The model under review builds one solid part; all positions refer to its coordinate system, in mm. A direction names the side the tool comes from. Give positions to 0.01 mm unless a question says otherwise; leave off trailing zeros. Loops run counter-clockwise (first coordinate to the right, second up) from the corner with the lowest first, then second, coordinate; pieces in that order, holes last. Notation, with made-up numbers: M -14,3.25 L 34,3.25 A15 cw 34,12.25 Z; hole C 39.5,77.5 d6. An arc over 180 degrees is marked long. Return JSON: item names as keys, results as strings.
```python
from build123d import *

# Parameters (mm, degrees)
BOSS_EXTRUDE1_DEPTH  = 10
FILLET1_R            = 1
SKETCH2_W            = 21.86553483
SKETCH2_H            = 30.5
CUT_EXTRUDE1_DEPTH   = 5
FILLET1_OF_MIRROR1_R = 1


with BuildPart() as part:
    # Sketch1 → Boss-Extrude1 (new body)
    with BuildSketch(Plane(origin=(0, 0, 0), x_dir=(1, 0, 0), z_dir=(0, 1, 0))):
        Polygon((-5, 57.097150921), (34.3, 57.097150921), (34.3, 55.097150921), (31.675, 55.097150921), (31.675, 52.597150921), (31.675, 2.599340873), (31.675, 0.099340873), (34.3, 0.099340873), (34.3, -4.5), (-5, -4.5), align=None)
        Polygon((-2.625, 45), (-2.625, 0), (-2.625, -2.5), (0, -2.5), (2.625, -2.5), (2.625, 0), (2.625, 45), (2.625, 47.5), (0, 47.5), (-2.625, 47.5), align=None, mode=Mode.SUBTRACT)
    boss_extrude1 = extrude(amount=BOSS_EXTRUDE1_DEPTH)

    # Fillet1
    fillet1_edges = [part.edges().sort_by_distance(p)[0] for p in [
        (31.675, 5, -55.097150921),
        (31.675, 5, -0.099340873),
        (-2.625, 5, -47.5),
        (-2.625, 5, 2.5),
        (2.625, 5, 2.5),
        (2.625, 5, -47.5),
    ]]
    fillet(fillet1_edges, radius=FILLET1_R)

    # Sketch2 → Cut-Extrude1 (cut)
    with BuildSketch(Plane(origin=(0, 10, 0), x_dir=(1, 0, 0), z_dir=(0, 1, 0))):
        with Locations((20.742232585, 23.8519351)):
            Rectangle(SKETCH2_W, SKETCH2_H)
    cut_extrude1 = extrude(amount=-CUT_EXTRUDE1_DEPTH, mode=Mode.SUBTRACT)

    # Mirror1: Boss-Extrude1, Cut-Extrude1 across plane
    add(boss_extrude1.mirror(Plane(origin=(34.3, 10, -0.099340873), x_dir=(0, 0, 1), z_dir=(-1, 0, 0))))
    add(cut_extrude1.mirror(Plane(origin=(34.3, 10, -0.099340873), x_dir=(0, 0, 1), z_dir=(-1, 0, 0))), mode=Mode.SUBTRACT)

    # Fillet1 of Mirror1
    fillet1_of_mirror1_edges = [part.edges().sort_by_distance(p)[0] for p in [
        (36.925, 5, -55.097150921),
        (36.925, 5, -0.099340873),
        (71.225, 5, -47.5),
        (71.225, 5, 2.5),
        (65.975, 5, 2.5),
        (65.975, 5, -47.5),
    ]]
    fillet(fillet1_of_mirror1_edges, radius=FILLET1_OF_MIRROR1_R)


solid = part.part
```
1) Wall thickness on L1, parallel to X at y = 8, z = -14.5 (3 decimals); L2, parallel to X at y = 4.75, z = -46 (3 decimals); L3, parallel to X at y = 9.75, z = 1 (3 decimals): over which ranges is each line inside the solid? List them lowest first. Write a range as from..to.
From the geometry:
{"L1": "-5..-2.625, 2.625..9.809, 58.791..65.975, 71.225..73.6", "L2": "-5..-2.625, 2.625..31.675, 36.925..65.975, 71.225..73.6", "L3": "-5..-2.625, 2.625..65.975, 71.225..73.6"}
2) The part is to be moulded in two halves that separate along Z. For faces 1 (the face through (2.625, 5, -23)), 2 (the face through (42, 0, -27)), 3 (the face through (34, 5, 4.5)), say which applies: released by +Z, released by -Z, zero draft, split by the parting line, or undercut.
From the geometry:
{"face 1": "undercut", "face 2": "zero draft", "face 3": "released by +Z"}
3) Insertion check: pin 1 (1 mm diameter, centred on x = 32, z = -22.5, fed in from +Y). The pin has a flat end and moves straight along its axis. Give the tip position at first contact, or say it passes through.
From the geometry:
{"pin 1": "y = 5"}
4) Consider section A-A on x = 0.5. Write out the cut boundary in (y, z).
From the geometry:
{"outline": "M 0,-57.1 L 10,-57.1 L 10,-47.5 L 0,-47.5 Z; M 0,2.5 L 10,2.5 L 10,4.5 L 0,4.5 Z"}
5) Consider section B-B on z = -36. Write out the cut boundary in (x, y) (3 decimals), then the cut area to 3 significant figures.
From the geometry:
{"outline": "M -5,0 L -2.625,0 L -2.625,10 L -5,10 Z; M 2.625,0 L 31.675,0 L 31.675,5 L 9.809,5 L 9.809,10 L 2.625,10 Z; M 36.925,0 L 65.975,0 L 65.975,10 L 58.791,10 L 58.791,5 L 36.925,5 Z; M 71.225,0 L 73.6,0 L 73.6,10 L 71.225,10 Z", "area": "410 mm²"}
6) Consider section D-D on y = 4. Write out the cut boundary in (x, z) (3 decimals), then the cut area to 3 significant figures.
From the geometry:
{"outline": "M -5,-57.097 L 73.6,-57.097 L 73.6,4.5 L -5,4.5 Z; hole M -2.625,-46.5 A1 ccw -1.625,-47.5 L 1.625,-47.5 A1 ccw 2.625,-46.5 L 2.625,1.5 A1 ccw 1.625,2.5 L -1.625,2.5 A1 ccw -2.625,1.5 Z; hole M 31.675,-54.097 A1 ccw 32.675,-55.097 L 35.925,-55.097 A1 ccw 36.925,-54.097 L 36.925,-1.099 A1 ccw 35.925,-0.099 L 32.675,-0.099 A1 ccw 31.675,-1.099 Z; hole M 65.975,-46.5 A1 ccw 66.975,-47.5 L 70.225,-47.5 A1 ccw 71.225,-46.5 L 71.225,1.5 A1 ccw 70.225,2.5 L 66.975,2.5 A1 ccw 65.975,1.5 Z", "area": "4,030 mm²"}
7) Tool access review of faces 4 (the face through (58.791, 8, -24)), 5 (the face through (69, 5, 2.5)), 6 (the face through (42, 10, -40)): name each direction out of +Z, -Z, +X, -X, +Y, -Y from which nothing blocks a thin tool from reaching the whole face with its end or side.
From the geometry:
{"face 4": "+Y", "face 5": "+Y, -Y", "face 6": "+Z, -Z, +X, -X, +Y"}
8) Consider section C-C on z = -51.5. Write out the cut boundary in (x, y) (3 decimals), then the cut area to 4 significant figures.
From the geometry:
{"outline": "M -5,0 L 31.675,0 L 31.675,10 L -5,10 Z; M 36.925,0 L 73.6,0 L 73.6,10 L 36.925,10 Z", "area": "733.5 mm²"}
